Verification items for this drawing (mm, ordinates from the low corner). Round coordinates to 2 decimals unless told otherwise and drop trailing zeros. Order: outer loops, then holes, each group sorted by start corner. A loop starts at its lowest first (then second) coordinate and runs counter-clockwise, first axis right, second up. Notation, with made-up numbers: (-31.75, 60.25) - (-11.75, 60.25) arc R30 cw to (-11.75, 85.25) - close; hole circle Ø2 at (-31.75, -4). An arc over 180 degrees is marked (long way). Return JSON: item names as keys, results as strings. Group by question number.
Q1. Sectioned sample at C-C, the plane z = 154. Record the cut outline in (x, y), then the cut area to 3 significant figures.
Q2. Material ranges on line 1 along Z through (x, y) = (15.5, 235.5); line 2 along Y through (x, z) = (17, 20.5); line 3 along Y through (x, z) = (16.25, 83) (1 decimal), recorded low to high.
Q3. Sectioned sample at B-B, the plane y = 226.5. Record the cut outline in (x, z).
Q4. Sectioned sample at A-A, the plane x = 16. Record the cut outline in (y, z) (1 decimal).
Q5. Gauge pin test, flat end, axial feed: pin 1 Ø6 at (x, z) = (14.5, 114) entering from -Y. Record the tip position at first contact, or that the pin passes through.
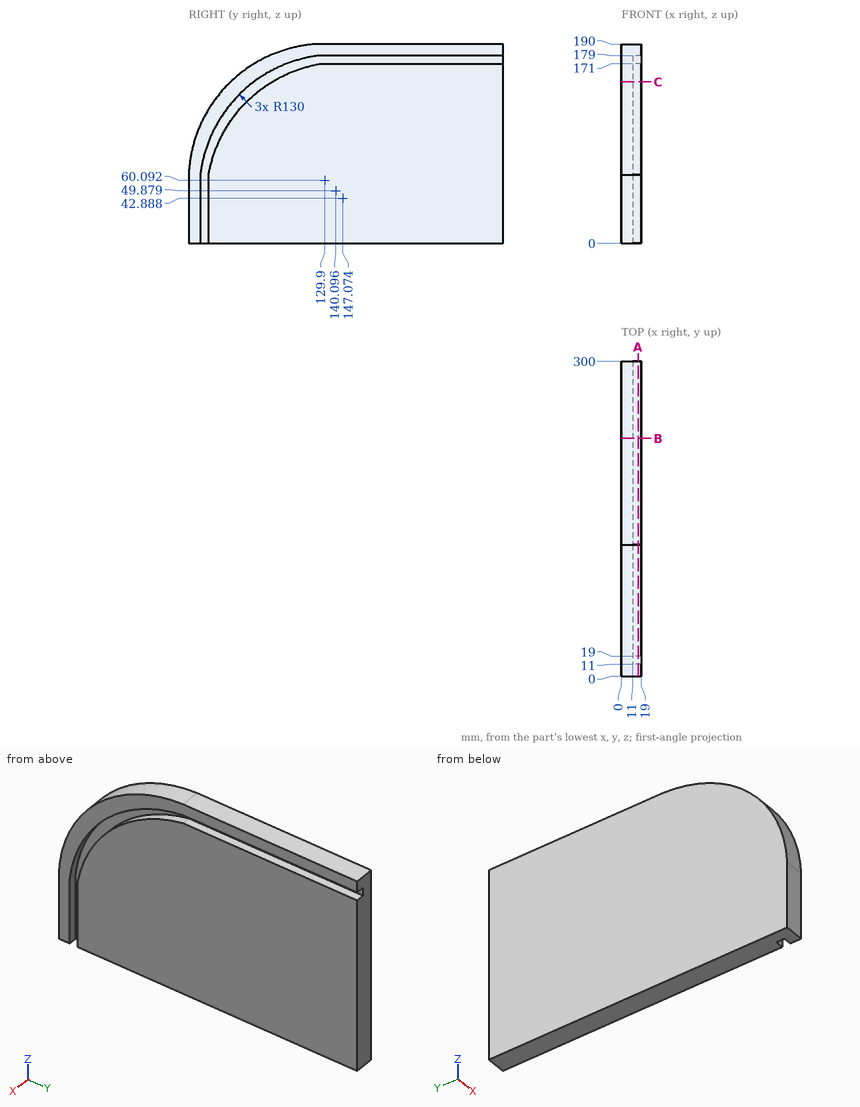
Reply:
{
 "1": {"outline": "(0, 40) - (19, 40) - (19, 62.26) - (11, 62.26) - (11, 79.59) - (19, 79.59) - (19, 300) - (0, 300) - close", "area": "4,800 mm^2"},
 "2": {"line 1": "0 to 171, 179 to 190", "line 2": "0 to 11, 19 to 300", "line 3": "1.9 to 14.4, 23.4 to 300"},
 "3": {"outline": "(0, 0) - (19, 0) - (19, 171) - (11, 171) - (11, 179) - (19, 179) - (19, 190) - (0, 190) - close"},
 "4": {"outline": "(0, 0) - (11, 0) - (11, 65.2) arc R130 cw to (125, 179) - (300, 179) - (300, 190) - (125, 190) arc R130 ccw to (0, 65.2) - close; (19, 0) - (300, 0) - (300, 171) - (125, 171) arc R130 ccw to (19, 65.2) - close"},
 "5": {"pin 1": "y = 10.28"}
}
